from build123d import *

# Parameters (mm, degrees)
BOX004_W          = 160
BOX004_H          = 100
BOX004_DEPTH      = 5
CYLINDER001_R     = 20
CYLINDER001_DEPTH = 3
BOX003_W          = 170
BOX003_H          = 110
BOX003_DEPTH      = 3


with BuildPart() as box004:
    # Box004 → Box004 (new body)
    with BuildSketch(Plane(origin=(5, 5, 3), x_dir=(1, 0, 0), z_dir=(0, 0, 1))):
        with Locations((80, 50)):
            Rectangle(BOX004_W, BOX004_H)
    extrude(amount=BOX004_DEPTH)


with BuildPart() as cilindro001:
    # Cylinder001 → Cylinder001 (new body)
    with BuildSketch(Plane(origin=(80, 0, 0), x_dir=(1, 0, 0), z_dir=(0, 0, 1))):
        Circle(CYLINDER001_R)
    extrude(amount=CYLINDER001_DEPTH)


with BuildPart() as obj1:
    # Box003 → Box003 (new body)
    with BuildSketch(Plane.XY):
        with Locations((85, 55)):
            Rectangle(BOX003_W, BOX003_H)
    extrude(amount=BOX003_DEPTH)

    # Fusion001: union Cilindro001
    add(cilindro001.part)


with BuildPart() as obj1_1:
    # Fusion001 placement: moved
    add(obj1.part.moved(Location((0, 0, 3))))

    # Cut004: cut Box004
    add(box004.part, mode=Mode.SUBTRACT)


with BuildPart() as obj1_2:
    # Cut004 placement: moved
    add(obj1_1.part.moved(Location((5, -30, 5))))


solid = obj1_2.part
Geometry check sheet. Reference: the model listing, model coordinates, mm. Round coordinates to 2 decimals unless told otherwise and drop trailing zeros. Loops run counter-clockwise (first coordinate to the right, second up) from the corner with the lowest first, then second, coordinate; pieces in that order, holes last.
Item 1: Gauge pin test, flat end, axial feed: pin 1 (0.9 mm diameter, centred on x = 40.5, z = 9, fed in from -Y). Record the tip position at first contact, or that the pin passes through.
Item 2: Cross-section at C-C on y = -12. Record the boundary of the cut face in (x, z).
Item 3: Cross-section at A-A on x = 73. Record the boundary of the cut face in (y, z).
Item 4: Cross-section at B-B on z = 10.3. Record the boundary of the cut face in (x, y).
Item 5: Thickness scan on line 1 (X direction, y = 26, z = 10.3); line 2 (Y direction, x = 32.5, z = 8.3); line 3 (Y direction, x = 98, z = 10.65). Record the ranges inside material, lowest first.
Answer sheet:
1. pin 1: stops at y = -30
2. outline: (5, 8) - (10, 8) - (10, 11) - (5, 11) - close; (170, 8) - (175, 8) - (175, 11) - (170, 11) - close
3. outline: (-46, 8) - (-25, 8) - (-25, 11) - (-46, 11) - close; (75, 8) - (80, 8) - (80, 11) - (75, 11) - close
4. outline: (5, -30) - (65, -30) arc R20 ccw to (105, -30) - (175, -30) - (175, 80) - (5, 80) - close; hole (10, -25) - (170, -25) - (170, 75) - (10, 75) - close
5. line 1: x = 5 to 10, 170 to 175
5. line 2: y = -30 to -25, 75 to 80
5. line 3: y = -45.2 to -25, 75 to 80
